The figure shows three views and two pictorial views of one solid part (mm, origin at its lowest corner). Answer the questions. A direction names the side the tool comes from. Coordinates: 2 decimals unless noted, no trailing zeros. Order: outer loops, then holes, each group sorted by start corner. A loop starts at its lowest first (then second) coordinate and runs counter-clockwise, first axis right, second up. Notation, with made-up numbers: (-15, -29.5) - (-1, -29.5) arc R35 ccw to (-1, 5.5) - close; hole circle Ø4 at (85.5, 4). An arc over 180 degrees is marked (long way). Use one line per item in the form item = value. Start each with the question number.
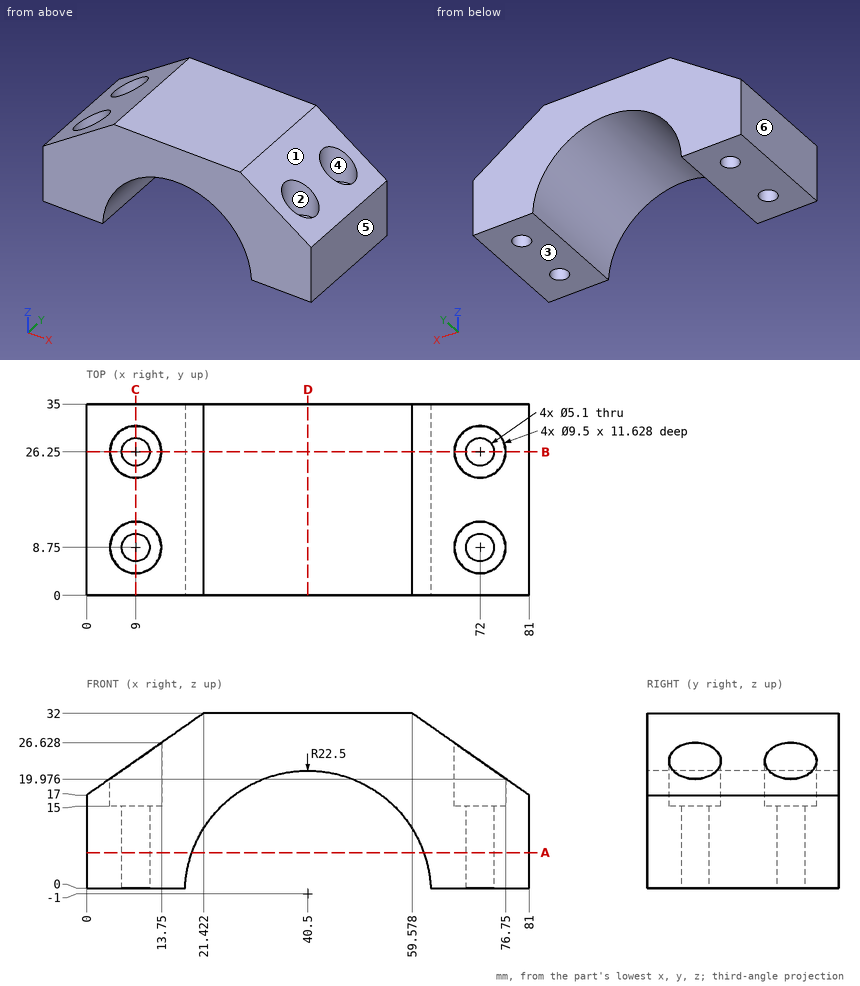
Q1. A cutting plane is placed at D-D (x = 40.5). Give the vertices of the cut face in (y, z).
Q2. A cutting plane is placed at B-B (y = 26.25). Give the vertices of the cut face in (x, z), then the cut area to 3 significant figures.
Q3. Consider probe 1 along Y at (x, z) = (9, 19); probe 2 along Y at (x, z) = (72, 9); probe 3 along X at (y, z) = (11, 4.5). Determine where each line is inside the solid, lowest interval first.
Q4. A cutting plane is placed at C-C (x = 9). Give the vertices of the cut face in (y, z).
Q5. For a pull along X with two mould halves and no side action, classify the marked faces 3, 4, 5 and 6 as +X half, -X half, draft (parallel to the pull), parting line (faces both ways), or undercut.
Q6. Which of the six approach directions +Z, -Z, +X, -X, +Y, -Y give full straight-line access (tool end or side, diameter ignored) to the marked faces 1 and 2?
Q7. Given P1, Ø8, axis at y = 11.5, z = 23.5, coming from the -X side; P2, Ø1, axis at x = 21, y = 31, coming from the -Z side; P3, Ø5.5, axis at x = 72, y = 8.75, coming from the -Z side; P4, Ø8, axis at x = 9, y = 26.25, coming from the +Z side, each flat-ended and moving along its own axis, determine where each tip first touches the part or whether it passes through.
Q8. A cutting plane is placed at A-A (z = 6.5). Give the vertices of the cut face in (x, y), then the cut area to 3 significant figures.
Result sheet:
q1.outline = (0, 21.5) - (35, 21.5) - (35, 32) - (0, 32) - close
q2.outline = (0, 0) - (6.45, 0) - (6.45, 15) - (4.25, 15) - (4.25, 19.98) - (0, 17) - close; (11.55, 0) - (18.02, 0) arc R22.5 cw to (62.98, 0) - (69.45, 0) - (69.45, 15) - (67.25, 15) - (67.25, 26.63) - (59.58, 32) - (21.42, 32) - (13.75, 26.63) - (13.75, 15) - (11.55, 15) - close; (74.55, 0) - (81, 0) - (81, 17) - (76.75, 19.98) - (76.75, 15) - (74.55, 15) - close
q2.area = 1,210 mm^2
q3.probe_1 = 0 to 4, 13.5 to 21.5, 31 to 35
q3.probe_2 = 0 to 6.2, 11.3 to 23.7, 28.8 to 35
q3.probe_3 = 0 to 7.8, 10.2 to 18.68, 62.32 to 70.8, 73.2 to 81
q4.outline = (0, 0) - (6.2, 0) - (6.2, 15) - (4, 15) - (4, 23.3) - (0, 23.3) - close; (11.3, 0) - (23.7, 0) - (23.7, 15) - (21.5, 15) - (21.5, 23.3) - (13.5, 23.3) - (13.5, 15) - (11.3, 15) - close; (28.8, 0) - (35, 0) - (35, 23.3) - (31, 23.3) - (31, 15) - (28.8, 15) - close
q5.face_3 = draft
q5.face_4 = undercut
q5.face_5 = +X half
q5.face_6 = -X half
q6.face_1 = +Z, +X, +Y, -Y
q6.face_2 = +Z
q7.P1 = 3.57
q7.P2 = 9.31
q7.P3 = 0
q7.P4 = 15
q8.outline = (0, 0) - (19.29, 0) - (19.29, 35) - (0, 35) - close; (61.71, 0) - (81, 0) - (81, 35) - (61.71, 35) - close; hole circle Ø5.1 at (9, 8.75); hole circle Ø5.1 at (9, 26.25); hole circle Ø5.1 at (72, 8.75); hole circle Ø5.1 at (72, 26.25)
q8.area = 1,270 mm^2
